from build123d import *

# Parameters (mm, degrees)
ESBO_O1_R                  = 4
RESSALTO_EXTRUS_O1_DEPTH   = 25
CORTE_EXTRUS_O1_DEPTH      = 38.749172176
CORTE_EXTRUS_O1_DEPTH_BACK = 38.749172176
ESBO_O2_W                  = 22
ESBO_O2_H                  = 15
ESBO_O3_R                  = 1.6
CORTE_EXTRUS_O2_DEPTH      = 20
RESSALTO_EXTRUS_O3_DEPTH   = 2


with BuildPart() as part:
    # Esboço1 → Ressalto-extrusão1 (new body)
    with BuildSketch(Plane.XY):
        with BuildLine():
            Line((0, 10), (-20, 10))
            Line((-20, 10), (-20, -10))
            Line((-20, -10), (0, -10))
            ThreePointArc((0, -10), (10, 0), (0, 10))
        make_face()
        Circle(ESBO_O1_R, mode=Mode.SUBTRACT)
    extrude(amount=RESSALTO_EXTRUS_O1_DEPTH)

    # Esboço2 → Corte-extrusão1 (cut, two sides: drawn at the far end of the back side and taken through both)
    with BuildSketch(Plane(origin=(0, 10, 0), x_dir=(1, 0, 0), z_dir=(0, 1, 0)).offset(-CORTE_EXTRUS_O1_DEPTH_BACK)):
        with Locations((-1, -7.5)):
            Rectangle(ESBO_O2_W, ESBO_O2_H)
    extrude(amount=CORTE_EXTRUS_O1_DEPTH + CORTE_EXTRUS_O1_DEPTH_BACK, mode=Mode.SUBTRACT)

    # Esboço3 → Corte-extrusão2 (cut)
    with BuildSketch(Plane(origin=(-12, 0, 0), x_dir=(0, 0, -1), z_dir=(1, 0, 0))):
        with Locations((-5, 0)):
            Circle(ESBO_O3_R)
    extrude(amount=-CORTE_EXTRUS_O2_DEPTH, mode=Mode.SUBTRACT)

    # Esboço5 → Ressalto-extrusão3 (add)
    with BuildSketch(Plane.XY.offset(25)):
        with BuildLine():
            Line((0, 10), (-20, 10))
            Line((-20, 10), (-20, -10))
            Line((-20, -10), (0, -10))
            ThreePointArc((0, -10), (10, 0), (0, 10))
        make_face()
    extrude(amount=RESSALTO_EXTRUS_O3_DEPTH)


solid = part.part
For this review, take the finished solid that the model builds, in its own axes (mm). A direction names the side the tool comes from. Coordinates: 2 decimals unless noted, no trailing zeros. Order: outer loops, then holes, each group sorted by start corner. A loop starts at its lowest first (then second) coordinate and runs counter-clockwise, first axis right, second up. Notation, with made-up numbers: (8.5, -16.75) - (59.5, -16.75) arc R17 ccw to (59.5, 7.25) - close; hole circle Ø4 at (-22.75, -22). An arc over 180 degrees is marked (long way). Answer as CSV lines item,"result". Start each with the question number.
1) Add section C-C (z = 23). State the section outline as (x, y) points, then the cut area to 3 significant figures.
2) To check wall thickness, follow line 1 along Y through (x, z) = (-13.5, 5); line 2 along X through (y, z) = (0, 19.25); line 3 along Z through (x, y) = (7, -0.25). State the ranges of each line that lie inside material, in increasing order. Write a range as [from, to].
3) Add section D-D (x = 3.5). State the section outline as (y, z) points.
4) Machinability: for faces 1 (the flat face through (-5, 0, 27)), 2 (the flat face through (0, 0, 25)), 3 (the flat face through (-4, 2, 15)), which of the approach directions +Z, -Z, +X, -X, +Y, -Y give a long, thin tool a straight path to every point of the face, cutting with its end or side? Answer none if there is none.
5) Insertion check: P1, Ø4, axis at x = -1.5, y = 0.5, coming from the -Z side; P2, Ø7.5, axis at y = 0, z = 6.5, coming from the +X side; P3, Ø2, axis at x = 5, z = 20, coming from the -Y side; P4, Ø1.9, axis at y = 0, z = 5, coming from the +X side. Each pin has a flat end and moves straight along its axis. Give the tip position at first contact, or say it passes through.
6) Add section B-B (z = 5). State the section outline as (x, y) points, then the cut area to 3 significant figures.
7) Draft analysis for pull direction Y (two halves, no side actions). For faces 4 (the cylindrical face through (-0.867, -3.905, 19.93)), 5 (the cylindrical face through (10, 0, 21)), 6 (the flat face through (-16, 0, 0)), 7 (the cylindrical face through (-15.94, 0.07, 6.6)), state which applies: +Y half, -Y half, draft (parallel to the pull), parting line (faces both ways), or undercut.
8) Add section A-A (y = 0). State the section outline as (x, z) points, then the cut area to 3 significant figures.
Result:
1,outline,"(-20, -10) - (0, -10) arc R10 ccw to (0, 10) - (-20, 10) - close; hole circle Ø8 at (0, 0)"
1,area,"507 mm^2"
2,line 1,"[-10, -1.6], [1.6, 10]"
2,line 2,"[-20, -4], [4, 10]"
2,line 3,"[15, 27]"
3,outline,"(-9.37, 15) - (-1.94, 15) - (-1.94, 25) - (1.94, 25) - (1.94, 15) - (9.37, 15) - (9.37, 27) - (-9.37, 27) - close"
4,face 1,"+Z, +X, -X, +Y, -Y"
4,face 2,"-Z"
4,face 3,"-Z, +X, +Y, -Y"
5,P1,"z = 25"
5,P2,"x = -12"
5,P3,"y = -9.17"
5,P4,"through"
6,outline,"(-20, -10) - (-12, -10) - (-12, -1.6) - (-20, -1.6) - close; (-20, 1.6) - (-12, 1.6) - (-12, 10) - (-20, 10) - close"
6,area,"134 mm^2"
7,face 4,"undercut"
7,face 5,"parting line"
7,face 6,"draft"
7,face 7,"undercut"
8,outline,"(-20, 0) - (-12, 0) - (-12, 3.4) - (-20, 3.4) - close; (-20, 6.6) - (-12, 6.6) - (-12, 15) - (-4, 15) - (-4, 25) - (4, 25) - (4, 15) - (10, 15) - (10, 27) - (-20, 27) - close"
8,area,"374 mm^2"
